Work out the finished part from the listing and answer in its coordinate system (mm). A direction names the side the tool comes from. Coordinates: 2 decimals unless noted, no trailing zeros. Loops run counter-clockwise (first coordinate to the right, second up) from the corner with the lowest first, then second, coordinate; pieces in that order, holes last. Notation, with made-up numbers: (-5, 32) -> (51, 32) arc R22 cw to (51, 54) -> close; hole circle Ø6 at (-1, -36.5). An arc over 180 degrees is marked (long way). Use a Markdown table: item, result.
from build123d import *

# Parameters (mm, degrees)
EXTRUDE_1_DEPTH          = 15
FILLET_1_R               = 30
SHELL_1_T                = -2
CUT_EXTRUDE_1_DEPTH      = 145.568322948
CUT_EXTRUDE_1_DEPTH_BACK = 145.568322948
SKETCH_3_W               = 2
SKETCH_3_H               = 1
SKETCH_3_W_2             = 1
SKETCH_3_H_2             = 3
CUT_EXTRUDE_2_DEPTH      = 3


with BuildPart() as part:
    # 草图1 → 拉伸-薄壁1 (new, symmetric)
    with BuildSketch(Plane(origin=(0, 0, 0), x_dir=(1, 0, 0), z_dir=(0, 1, 0))):
        Polygon((0, 100), (0, 0), (100, 0), (100, -30), (-30, -30), (-30, 100), align=None)
    extrude(amount=EXTRUDE_1_DEPTH, both=True)

    # 圆角1
    fillet_1_edges = [part.edges().sort_by_distance(p)[0] for p in [
        (-30, 0, 30),
    ]]
    fillet(fillet_1_edges, radius=FILLET_1_R)

    # 抽壳1
    shell_1_openings = [part.faces().sort_by_distance(p)[0] for p in [
        (100, 0, 15),
        (-15, 0, -100),
    ]]
    offset(amount=SHELL_1_T, openings=shell_1_openings, kind=Kind.INTERSECTION)

    # 草图2 → 切除-拉伸1 (cut, two sides: drawn at the far end of the back side and taken through both)
    with BuildSketch(Plane(origin=(0, 15, 0), x_dir=(1, 0, 0), z_dir=(0, 1, 0)).offset(-CUT_EXTRUDE_1_DEPTH_BACK)):
        with BuildLine():
            ThreePointArc((-28, 0), (-19.798989873, -19.798989873), (0, -28))
            Line((0, -28), (0, -27))
            ThreePointArc((0, -27), (-19.091883092, -19.091883092), (-27, 0))
            Line((-27, 0), (0, 0))
            Line((0, 0), (0, 1))
            Line((0, 1), (-28, 1))
            Line((-28, 1), (-28, 0))
        make_face()
    extrude(amount=CUT_EXTRUDE_1_DEPTH + CUT_EXTRUDE_1_DEPTH_BACK, mode=Mode.SUBTRACT)

    # 草图3 → 切除-拉伸2 (cut)
    with BuildSketch(Plane(origin=(0, 15, 0), x_dir=(1, 0, 0), z_dir=(0, 1, 0))):
        with Locations((-29, 0.5)):
            Rectangle(SKETCH_3_W, SKETCH_3_H)
        with Locations((0.5, -28.5)):
            Rectangle(SKETCH_3_W_2, SKETCH_3_H_2)
    cut_extrude_2 = extrude(amount=-CUT_EXTRUDE_2_DEPTH, mode=Mode.SUBTRACT)

    # 镜向1: 切除-拉伸2 across plane
    add(cut_extrude_2.mirror(Plane.ZX), mode=Mode.SUBTRACT)


solid = part.part
Q1. Given pin 1 Ø0.5 at (x, y) = (0.5, -14) entering from +Z; pin 2 Ø8 at (y, z) = (5, -74.5) entering from +X; pin 3 Ø3.5 at (y, z) = (13, 29) entering from -X; pin 4 Ø1.1 at (x, z) = (-28.5, -0.5) entering from -Y, each flat-ended and moving along its own axis, determine where each tip first touches the part or whether it passes through.
Solved:
| item | result |
|---|---|
| pin 1 | z = 27 |
| pin 2 | x = 0 |
| pin 3 | x = -12.55 |
| pin 4 | y = -15 |
Q2. Section D-D on z = -52.5 is taken. Determine the outline of the cut face in (x, y), and give its area (3 significant figures).
Solved:
| item | result |
|---|---|
| outline | (-30, -15) -> (0, -15) -> (0, 15) -> (-30, 15) -> close; hole (-28, -13) -> (-2, -13) -> (-2, 13) -> (-28, 13) -> close |
| area | 224 mm² |
Q3. Section B-B on x = 45 is taken. Determine the outline of the cut face in (y, z), and give its area (3 significant figures).
Solved:
| item | result |
|---|---|
| outline | (-15, 0) -> (15, 0) -> (15, 30) -> (-15, 30) -> close; hole (-13, 2) -> (13, 2) -> (13, 28) -> (-13, 28) -> close |
| area | 224 mm² |
Q4. For faces 1 (the flat face through (48, 0, 2)), 2 (the flat face through (1, 14, 29)), 3 (the flat face through (-15, 13, -51)), determine the directions among +Z, -Z, +X, -X, +Y, -Y from which every point of the face is accessible in a straight line to the end or side of a thin tool.
Solved:
| item | result |
|---|---|
| face 1 | +X |
| face 2 | +Z, +Y |
| face 3 | -Z |
Q5. Section A-A on y = -2.25 is taken. Determine the outline of the cut face in (x, z).
Solved:
| item | result |
|---|---|
| outline | (-30, -100) -> (-28, -100) -> (-28, 0) arc R28 cw to (0, 28) -> (100, 28) -> (100, 30) -> (0, 30) arc R30 ccw to (-30, 0) -> close; (-2, -100) -> (0, -100) -> (0, -1) -> (-2, -1) -> close; (-2, 0) -> (100, 0) -> (100, 2) -> (-2, 2) -> close |
Q6. Section C-C on z = 22.5 is taken. Determine the outline of the cut face in (x, y), and give its area (3 significant figures).
Solved:
| item | result |
|---|---|
| outline | (-19.84, -15) -> (-16.67, -15) -> (-16.67, 15) -> (-19.84, 15) -> close; (-14.92, -15) -> (100, -15) -> (100, -13) -> (-14.92, -13) -> close; (-14.92, 13) -> (100, 13) -> (100, 15) -> (-14.92, 15) -> close |
| area | 555 mm² |
Q7. Determine the mould class of faces 4 (the flat face through (-28, 0, -51)), 5 (the cylindrical face through (-20.015, -0.21, 19.58)), 6 (the flat face through (37, 15, 15)), 7 (the flat face through (-19.4, -15, 20.5)) for opening direction Y: pulls with the +Y half, pulls with the -Y half, needs draft (parallel to the pull), parting line crosses it, or undercut.
Solved:
| item | result |
|---|---|
| face 4 | undercut |
| face 5 | needs draft |
| face 6 | pulls with the +Y half |
| face 7 | pulls with the -Y half |
Q8. Consider line 1 (Y direction, x = 70.5, z = 15); line 2 (X direction, y = -8, z = -16); line 3 (Z direction, x = 12, y = 5). Determine where each line is inside the solid, lowest interval first. Write a range as [from, to].
Solved:
| item | result |
|---|---|
| line 1 | [-15, -13], [13, 15] |
| line 2 | [-30, -28], [-2, 0] |
| line 3 | [0, 2], [28, 30] |
